Could you check a few things on this model? Use its own coordinates, in mm. A direction names the side the tool comes from. Give positions to 0.01 mm unless a question says otherwise; leave off trailing zeros. Loops run counter-clockwise (first coordinate to the right, second up) from the corner with the lowest first, then second, coordinate; pieces in that order, holes last. Notation, with made-up numbers: M 7.25,22 L 29.25,22 A28 cw 29.25,43 Z; hole C 78,-18.75 d8. An arc over 180 degrees is marked long. Use a Markdown table: item, result. Add a question column.
1) We'd pull the mould along X, two halves only. Please class faces 1 (the flat face through (-48, 22, 13)), 2 (the cylindrical face through (-1.12, -23.884, 20.355)), 3 (the flat face through (50, -22, 3.9)): +X half, -X half, draft (parallel to the pull), parting line (faces both ways), or undercut.
2) If I drill on line 1 along Y through (x, z) = (-43, 18.5); line 2 along X through (y, z) = (-23, 4.5); line 3 along Y through (x, z) = (45.5, 20), over which ranges is the centre line in solid material (lowest first)? Write a range as [from, to].
3) Will this pin go through, and if not, where does the flat tip stop? pin 1 Ø4.5 at (x, z) = (72.3, 28.2) entering from -Y.
4) Suppose I cut it at C-C on z = 8.4. Count the separate pieces of the cut face and the enclosed holes in it, and give its area (3 significant figures).
5) Which directions (+Z, -Z, +X, -X, +Y, -Y) give clear straight access to the entire face, cutting with the end or side of a thin tool? Please do faces 4 (the flat face through (-50, 22, 22.9)), 5 (the cylindrical face through (33.5, -24.2, 13.27)).
6) Suppose I cut it at D-D on y = -7.5. List the corners of the cut face in (x, z) for me.
7) Suppose I cut it at B-B on x = 19.5. List the corners of the cut face in (y, z) for me.
8) Suppose I cut it at A-A on x = 45. List the corners of the cut face in (y, z) for me.
```python
from build123d import *

# Parameters (mm, degrees)
SKETCH1_W               = 160
SKETCH1_H               = 56
BOSS_EXTRUDE1_DEPTH     = 35
SKETCH2_W               = 32
SKETCH2_H               = 41
CUT_EXTRUDE1_DEPTH      = 167.159561868
FILLET1_R               = 5
SKETCH6_W               = 4
SKETCH6_H               = 19
CUT_EXTRUDE4_DEPTH      = 3
MIRROR4_COPY_1_SKETCH_W = 4
MIRROR4_COPY_1_SKETCH_H = 19
MIRROR4_COPY_1_DEPTH    = 3
SKETCH8_R               = 2.05
CUT_EXTRUDE6_DEPTH      = 167.159561868
SKETCH9_R               = 2.05
CUT_EXTRUDE7_DEPTH      = 104.735239914
SKETCH10_R              = 3
SKETCH10_R_2            = 1.5
BOSS_EXTRUDE3_DEPTH     = 10
SKETCH13_R              = 1.5
CUT_EXTRUDE9_DEPTH      = 96.431913025


with BuildPart() as part:
    # Sketch1 → Boss-Extrude1 (new body)
    with BuildSketch(Plane.XY):
        Rectangle(SKETCH1_W, SKETCH1_H)
    extrude(amount=BOSS_EXTRUDE1_DEPTH)

    # Sketch2 → Cut-Extrude1 (cut, through all)
    with BuildSketch(Plane.ZY.offset(80)):
        with Locations((19, 0)):
            Rectangle(SKETCH2_W, SKETCH2_H)
    extrude(amount=-CUT_EXTRUDE1_DEPTH, mode=Mode.SUBTRACT)

    # Fillet1
    fillet1_edges = [part.edges().sort_by_distance(p)[0] for p in [
        (0, -28, 0),
        (0, 28, 0),
    ]]
    fillet(fillet1_edges, radius=FILLET1_R)

    # Sketch6 → Cut-Extrude4 (cut)
    with BuildSketch(Plane.XZ.offset(-20.5)):
        with Locations((-50, 13.4)):
            Rectangle(SKETCH6_W, SKETCH6_H)
    cut_extrude4 = extrude(amount=-CUT_EXTRUDE4_DEPTH, mode=Mode.SUBTRACT)

    # Mirror3: Cut-Extrude4 across plane
    add(cut_extrude4.mirror(Plane.ZY), mode=Mode.SUBTRACT)

    # Mirror4: Cut-Extrude4 across plane
    add(cut_extrude4.mirror(Plane.ZX), mode=Mode.SUBTRACT)

    # Mirror4 copy 1 sketch → Mirror4 copy 1 (cut)
    with BuildSketch(Plane(origin=(0, -20.5, 0), x_dir=(-1, 0, 0), z_dir=(0, 1, 0))):
        with Locations((-50, 13.4)):
            Rectangle(MIRROR4_COPY_1_SKETCH_W, MIRROR4_COPY_1_SKETCH_H)
    extrude(amount=-MIRROR4_COPY_1_DEPTH, mode=Mode.SUBTRACT)

    # Sketch8 → Cut-Extrude6 (cut, through all)
    with BuildSketch(Plane.ZY.offset(80)):
        with Locations((18.4, -24.5)):
            Circle(SKETCH8_R)
        with Locations((8.4, -24.5)):
            Circle(SKETCH8_R)
    cut_extrude6 = extrude(amount=-CUT_EXTRUDE6_DEPTH, mode=Mode.SUBTRACT)

    # Mirror5: Cut-Extrude6 across plane
    add(cut_extrude6.mirror(Plane.ZX), mode=Mode.SUBTRACT)

    # Sketch9 → Cut-Extrude7 (cut, through all)
    with BuildSketch(Plane(origin=(0, 28, 0), x_dir=(1, 0, 0), z_dir=(0, 1, 0))):
        with Locations(Location((41.410879364, -25.216075278, 0), (0, 0, 270))):
            Circle(SKETCH9_R)
        with Locations(Location((33.410879423, -15.320010713, 0), (0, 0, 270))):
            Circle(SKETCH9_R)
        with Locations(Location((72.304393308, -28.203284125, 0), (0, 0, 270))):
            Circle(SKETCH9_R)
        with Locations(Location((-32.610879423, -15.320010713, 0), (0, 0, 270))):
            Circle(SKETCH9_R)
        with Locations(Location((-40.610879364, -25.216075278, 0), (0, 0, 270))):
            Circle(SKETCH9_R)
        with Locations(Location((-71.504393308, -28.203284125, 0), (0, 0, 270))):
            Circle(SKETCH9_R)
    extrude(amount=-CUT_EXTRUDE7_DEPTH, mode=Mode.SUBTRACT)

    # Sketch10 → Boss-Extrude3 (add)
    with BuildSketch(Plane(origin=(0, -20.5, 0), x_dir=(1, 0, 0), z_dir=(0, 1, 0))):
        with Locations(Location((-45, -13.4, 0), (0, 0, 180))):
            Circle(SKETCH10_R)
        with Locations(Location((-45, -13.4, 0), (0, 0, 270))):
            Circle(SKETCH10_R_2, mode=Mode.SUBTRACT)
    boss_extrude3 = extrude(amount=BOSS_EXTRUDE3_DEPTH)

    # Sketch13 → Cut-Extrude9 (cut, through all)
    with BuildSketch(Plane(origin=(0, -10.5, 0), x_dir=(1, 0, 0), z_dir=(0, 1, 0))):
        with Locations(Location((-45, -13.4, 0), (0, 0, 270))):
            Circle(SKETCH13_R)
    cut_extrude9 = extrude(amount=-CUT_EXTRUDE9_DEPTH, mode=Mode.SUBTRACT)

    # Mirror6: Boss-Extrude3, Cut-Extrude9 across plane
    add(boss_extrude3.mirror(Plane.ZY))
    add(cut_extrude9.mirror(Plane.ZY), mode=Mode.SUBTRACT)


solid = part.part
```
Answer block:
| question | item | result |
|---|---|---|
| 1 | face 1 | undercut |
| 1 | face 2 | draft |
| 1 | face 3 | undercut |
| 2 | line 1 | y = [-28, -26.55], [-22.45, -20.5], [20.5, 22.45], [26.55, 28] |
| 2 | line 2 | x = [-80, -52], [-48, 48], [52, 80] |
| 2 | line 3 | y = [-28, -25.78], [-23.22, -20.5], [20.5, 23.22], [25.78, 28] |
| 3 | pin 1 | stops at y = -28 |
| 4 | separate pieces | 8 |
| 4 | enclosed holes | 0 |
| 4 | area | 1,060 mm^2 |
| 5 | face 4 | none |
| 5 | face 5 | +Y, -Y |
| 6 | outline | M -80,0 L 80,0 L 80,3 L -80,3 Z |
| 7 | outline | M -28,5 A5 ccw -23,0 L 23,0 A5 ccw 28,5 L 28,35 L 20.5,35 L 20.5,3 L -20.5,3 L -20.5,35 L -28,35 Z; hole C -24.5,8.4 d4.1; hole C -24.5,18.4 d4.1; hole C 24.5,8.4 d4.1; hole C 24.5,18.4 d4.1 |
| 8 | outline | M -28,5 A5 ccw -23,0 L 23,0 A5 ccw 28,5 L 28,35 L 20.5,35 L 20.5,3 L -20.5,3 L -20.5,10.4 L -10.5,10.4 L -10.5,11.9 L -28,11.9 Z; M -28,14.9 L -10.5,14.9 L -10.5,16.4 L -20.5,16.4 L -20.5,35 L -28,35 Z; hole C -24.5,8.4 d4.1; hole C -24.5,18.4 d4.1; hole C 24.5,8.4 d4.1; hole C 24.5,18.4 d4.1 |
